```python
from build123d import *

# Parameters (mm, degrees)
SKETCH1_W           = 38.1
SKETCH1_H           = 25.4
BOSS_EXTRUDE1_DEPTH = 5
SKETCH3_R           = 7.25
SKETCH3_R_2         = 4.25
BOSS_EXTRUDE2_DEPTH = 32
SKETCH4_R           = 3.5
CUT_EXTRUDE1_DEPTH  = 44.047479384
CUT_EXTRUDE2_START  = -18
CUT_EXTRUDE2_DEPTH  = 18
BOSS_EXTRUDE3_START = -13
BOSS_EXTRUDE3_DEPTH = 13
SKETCH9_R           = 1.15
BOSS_EXTRUDE4_DEPTH = 6.21


with BuildPart() as part:
    # Sketch1 → Boss-Extrude1 (new body)
    with BuildSketch(Plane(origin=(0, 0, 0), x_dir=(1, 0, 0), z_dir=(0, 1, 0))):
        with Locations((-6.79173913, 0)):
            Rectangle(SKETCH1_W, SKETCH1_H)
    extrude(amount=BOSS_EXTRUDE1_DEPTH)

    # Sketch3 → Boss-Extrude2 (add)
    with BuildSketch(Plane(origin=(0, 5, 0), x_dir=(1, 0, 0), z_dir=(0, 1, 0))):
        with Locations(Location((-6.79173913, 0, 0), (0, 0, 270))):
            Circle(SKETCH3_R)
        with Locations(Location((-6.79173913, 0, 0), (0, 0, 270))):
            Circle(SKETCH3_R_2, mode=Mode.SUBTRACT)
    extrude(amount=BOSS_EXTRUDE2_DEPTH)

    # Sketch4 → Cut-Extrude1 (cut, through all)
    with BuildSketch(Plane(origin=(0, 5, 0), x_dir=(1, 0, 0), z_dir=(0, 1, 0))):
        with Locations(Location((7.17826087, 0, 0), (0, 0, 270))):
            Circle(SKETCH4_R)
        with Locations(Location((-20.76173913, 0, 0), (0, 0, 270))):
            Circle(SKETCH4_R)
    extrude(amount=-CUT_EXTRUDE1_DEPTH, mode=Mode.SUBTRACT)

    # Sketch6 → Cut-Extrude2 (cut)
    with BuildSketch(Plane(origin=(0, 37, 0), x_dir=(1, 0, 0), z_dir=(0, 1, 0)).offset(CUT_EXTRUDE2_START)):
        with BuildLine():
            Line((-3.117504516, 6.25), (-10.465973745, 6.25))
            ThreePointArc((-10.465973745, 6.25), (-6.79173913, 7.25), (-3.117504516, 6.25))
        make_face()
    extrude(amount=CUT_EXTRUDE2_DEPTH, mode=Mode.SUBTRACT)

    # Sketch8 → Boss-Extrude3 (add)
    with BuildSketch(Plane(origin=(0, 37, 0), x_dir=(1, 0, 0), z_dir=(0, 1, 0)).offset(BOSS_EXTRUDE3_START)):
        with BuildLine():
            Line((-14.04173913, 6.25), (-10.465973745, 6.25))
            ThreePointArc((-10.465973745, 6.25), (-13.084620067, 3.600298533), (-14.04173913, 0))
            Line((-14.04173913, 0), (-14.04173913, 6.25))
        make_face()
        with BuildLine():
            Line((0.45826087, 0), (0.45826087, 6.25))
            Line((0.45826087, 6.25), (-3.117504516, 6.25))
            ThreePointArc((-3.117504516, 6.25), (-0.498858194, 3.600298533), (0.45826087, 0))
        make_face()
    extrude(amount=BOSS_EXTRUDE3_DEPTH)

    # Sketch9 → Boss-Extrude4 (add)
    with BuildSketch(Plane(origin=(0, 0, -6.25), x_dir=(-1, 0, 0), z_dir=(0, 0, -1))):
        with Locations(Location((2.04173913, 30.5, 0), (0, 0, 180))):
            Circle(SKETCH9_R)
        with Locations(Location((11.54173913, 30.5, 0), (0, 0, 180))):
            Circle(SKETCH9_R)
    extrude(amount=BOSS_EXTRUDE4_DEPTH)


solid = part.part
```
Verification items for the finished model (mm, model axes). A direction names the side the tool comes from. Give positions to 0.01 mm unless a question says otherwise; leave off trailing zeros. Order: outer loops, then holes, each group sorted by start corner. A loop starts at its lowest first (then second) coordinate and runs counter-clockwise, first axis right, second up. Notation, with made-up numbers: M 14.25,42.25 L 24.25,42.25 A12 ccw 24.25,61.25 Z; hole C 58.25,-21.75 d8. An arc over 180 degrees is marked long. Answer in a Markdown table with one row per item. Add a question column.
Item 1: Gauge pin test, flat ends, axial feed: pin 1 (0.7 mm diameter, centred on x = -2.5, y = 30.5, fed in from -Z); pin 2 (5 mm diameter, centred on y = 28, z = -3, fed in from -X); pin 3 (6 mm diameter, centred on y = 28, z = 7, fed in from +X); pin 4 (5.5 mm diameter, centred on x = -20.76, z = 0, fed in from +Y). Record the tip position at first contact, or that the pin passes through.
Item 2: Section check D-D, the plane z = 4.75. Enter the section's corners in (x, y), and give its area (3 significant figures).
Item 3: Tool access check on faces 1 (the cylindrical face through (-10.562, 20.776, 1.961)), 2 (the flat face through (-2, 30, -12.46)), 3 (the flat face through (-1, 24, -5)), 4 (the flat face through (-14.042, 30, -3)), 5 (the cylindrical face through (-2.291, 31.623, -9.312)). Record the directions out of +Z, -Z, +X, -X, +Y, -Y that give a thin tool (end or side, any length) a straight path to the whole face; none if there is none.
Item 4: Section check A-A, the plane z = -9.25. Enter the section's corners in (x, y), and give its area (3 significant figures).
Item 5: Section check C-C, the plane y = 30.5. Enter the section's corners in (x, z), and give its area (3 significant figures).
Item 6: Scan lines: probe 1 along X at (y, z) = (1.45, 0); probe 2 along Y at (x, z) = (0, -4.5); probe 3 along X at (y, z) = (24.5, -0.25). Record each from-to range of solid material in increasing order. Write a range as from..to.
Item 7: Section check B-B, the plane x = -19.5. Enter the section's corners in (y, z), and give its area (3 significant figures).
Item 8: Mould release check, pull along Z, two halves, no side actions. Record for faces 6 (the cylindrical face through (-17.292, 2.535, -0.456)), 7 (the flat face through (-7, 2, 12.7)), 8 (the flat face through (-7, 0, 0)), 9 (the flat face through (-7, 2, -12.7)): released by +Z, released by -Z, zero draft, split by the parting line, or undercut.
Filled sheet:
| question | item | result |
|---|---|---|
| 1 | pin 1 | stops at z = -12.46 |
| 1 | pin 2 | stops at x = -14.04 |
| 1 | pin 3 | stops at x = -0.75 |
| 1 | pin 4 | passes through |
| 2 | outline | M -25.84,0 L 12.26,0 L 12.26,5 L -1.31,5 L -1.31,37 L -12.27,37 L -12.27,5 L -25.84,5 Z |
| 2 | area | 541 mm^2 |
| 3 | face 1 | +Y |
| 3 | face 2 | -Z, +X, -X, +Y |
| 3 | face 3 | -Z, +X |
| 3 | face 4 | +Z, -Z, -X, +Y |
| 3 | face 5 | -Z |
| 4 | outline | M -25.84,0 L 12.26,0 L 12.26,5 L -25.84,5 Z; C -11.54,30.5 d2.3; C -2.04,30.5 d2.3 |
| 4 | area | 199 mm^2 |
| 5 | outline | M -14.04,-6.25 L -12.69,-6.25 L -12.69,-12.46 L -10.39,-12.46 L -10.39,-6.25 L -3.19,-6.25 L -3.19,-12.46 L -0.89,-12.46 L -0.89,-6.25 L 0.46,-6.25 L 0.46,0 A7.25 ccw -14.04,0 Z; hole C -6.79,0 d8.5 |
| 5 | area | 145 mm^2 |
| 6 | probe 1 | x = -25.84..-24.26, -17.26..3.68, 10.68..12.26 |
| 6 | probe 2 | y = 0..5, 24..37 |
| 6 | probe 3 | x = -14.04..-11.03, -2.55..0.46 |
| 7 | outline | M 0,-12.7 L 5,-12.7 L 5,-3.26 L 0,-3.26 Z; M 0,3.26 L 5,3.26 L 5,12.7 L 0,12.7 Z |
| 7 | area | 94.4 mm^2 |
| 8 | face 6 | undercut |
| 8 | face 7 | released by +Z |
| 8 | face 8 | zero draft |
| 8 | face 9 | released by -Z |
